```python
from build123d import *

# Parameters (mm, degrees)
BOSS_EXTRUDE1_DEPTH          = 6
M5X0_8_TAPPED_HOLE1_D        = 4.2
F_4_0_4_DIAMETER_HOLE1_D     = 4
F_4_0_4_DIAMETER_HOLE1_DEPTH = 10
F_4_0_4_DIAMETER_HOLE1_TIP   = 1.201721238


with BuildPart() as part:
    # Sketch2 → Boss-Extrude1 (new body)
    with BuildSketch(Plane(origin=(0, 0, 0), x_dir=(1, 0, 0), z_dir=(0, 1, 0))):
        with BuildLine():
            Line((-12, -15), (12, -15))
            ThreePointArc((12, -15), (14.121320344, -14.121320344), (15, -12))
            Line((15, -12), (15, 12))
            ThreePointArc((15, 12), (14.121320344, 14.121320344), (12, 15))
            Line((12, 15), (-12, 15))
            ThreePointArc((-12, 15), (-14.121320344, 14.121320344), (-15, 12))
            Line((-15, 12), (-15, -12))
            ThreePointArc((-15, -12), (-14.121320344, -14.121320344), (-12, -15))
        make_face()
    extrude(amount=-BOSS_EXTRUDE1_DEPTH)

    # M5x0.8 Tapped Hole1 (through all)
    with Locations(Plane(origin=(0, 0, 0), x_dir=(1, 0, 0), z_dir=(0, 1, 0))):
        with Locations((0, 0), (0, 9), (0, -9)):
            Hole(M5X0_8_TAPPED_HOLE1_D / 2)

    # Ø4.0 (4) Diameter Hole1
    with Locations(Plane(origin=(0, 0, 0), x_dir=(1, 0, 0), z_dir=(0, 1, 0))):
        with Locations((-11.5, -11.5), (-11.5, 11.5), (11.5, 11.5), (11.5, -11.5)):
            Hole(F_4_0_4_DIAMETER_HOLE1_D / 2, depth=F_4_0_4_DIAMETER_HOLE1_DEPTH)
            with Locations((0, 0, -(F_4_0_4_DIAMETER_HOLE1_DEPTH + F_4_0_4_DIAMETER_HOLE1_TIP / 2))):  # 118° drill point
                Cone(0, F_4_0_4_DIAMETER_HOLE1_D / 2, F_4_0_4_DIAMETER_HOLE1_TIP, mode=Mode.SUBTRACT)


solid = part.part
```
CAD build for the part. Positions are in the model's coordinates, mm. Coordinates: 2 decimals unless noted, no trailing zeros. Loops run counter-clockwise (first coordinate to the right, second up) from the corner with the lowest first, then second, coordinate; pieces in that order, holes last. Notation, with made-up numbers: (-35, 73) - (0, 73) arc R29 cw to (0, 112) - close; hole circle Ø2 at (-2.75, 67.25). An arc over 180 degrees is marked (long way). Use CSV: the item, a comma, the result in double quotes. Start each with the question number.
Q1. Cut at B-B, the plane x = -11.5. List the corners of the cut face in (y, z).
Q2. Drop flat-ended pins along their axis: P1, Ø2.5, axis at x = 0, z = 0, coming from the +Y side; P2, Ø6.5, axis at x = -11.5, z = -11.5, coming from the +Y side. Give the stop position or say it passes through.
Q3. Cut at C-C, the plane x = 0. List the corners of the cut face in (y, z).
Q4. Cut at A-A, the plane z = 11.5. List the corners of the cut face in (x, y), then the cut area to 3 significant figures.
Q5. Probe probe 1 along X at (y, z) = (-2.8, -11.5); probe 2 along Z at (x, y) = (0, -3.4). List the from-to ranges inside material, lowest first. Write a range as from..to.
Q6. Two-plate mould, pull along Z, no slides. Class faces 1 (the cylindrical face through (14.14, -2.96, -14.1)), 2 (the flat face through (0, -3, 15)), 3 (the cylindrical face through (0.273, -3.042, -11.082)), 4 (the flat face through (0, -6, 3)): +Z half, -Z half, draft (parallel to the pull), parting line (faces both ways), or undercut.
Q7. Cut at D-D, the plane y = -4.05. List the corners of the cut face in (x, z).
Here are the results:
1,outline,"(-6, -15) - (0, -15) - (0, -13.5) - (-6, -13.5) - close; (-6, -9.5) - (0, -9.5) - (0, 9.5) - (-6, 9.5) - close; (-6, 13.5) - (0, 13.5) - (0, 15) - (-6, 15) - close"
2,P1,"through"
2,P2,"y = 0"
3,outline,"(-6, -15) - (0, -15) - (0, -11.1) - (-6, -11.1) - close; (-6, -6.9) - (0, -6.9) - (0, -2.1) - (-6, -2.1) - close; (-6, 2.1) - (0, 2.1) - (0, 6.9) - (-6, 6.9) - close; (-6, 11.1) - (0, 11.1) - (0, 15) - (-6, 15) - close"
4,outline,"(-15, -6) - (-13.5, -6) - (-13.5, 0) - (-15, 0) - close; (-9.5, -6) - (9.5, -6) - (9.5, 0) - (-9.5, 0) - close; (13.5, -6) - (15, -6) - (15, 0) - (13.5, 0) - close"
4,area,"132 mm2"
5,probe 1,"-15..-13.5, -9.5..9.5, 13.5..15"
5,probe 2,"-15..-11.1, -6.9..-2.1, 2.1..6.9, 11.1..15"
6,face 1,"-Z half"
6,face 2,"+Z half"
6,face 3,"undercut"
6,face 4,"draft"
7,outline,"(-15, -12) arc R3 ccw to (-12, -15) - (12, -15) arc R3 ccw to (15, -12) - (15, 12) arc R3 ccw to (12, 15) - (-12, 15) arc R3 ccw to (-15, 12) - close; hole circle Ø4 at (-11.5, -11.5); hole circle Ø4 at (-11.5, 11.5); hole circle Ø4.2 at (0, -9); hole circle Ø4.2 at (0, 0); hole circle Ø4.2 at (0, 9); hole circle Ø4 at (11.5, -11.5); hole circle Ø4 at (11.5, 11.5)"
